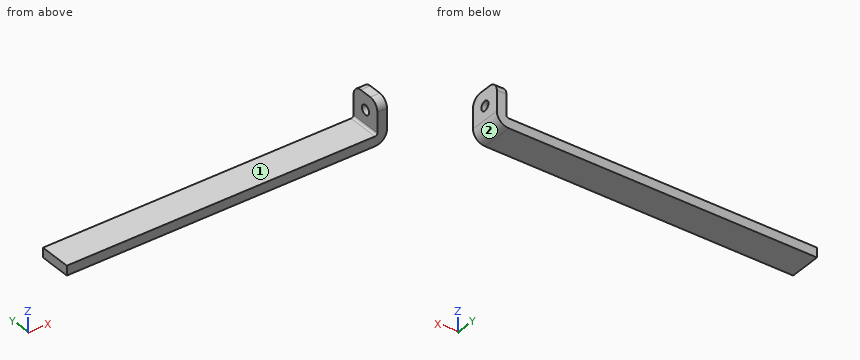
```python
from build123d import *

# Parameters (mm, degrees)
SKETCH_1_W                       = 100
SKETCH_1_H                       = 10
SM_BASE_FLANGE_1_DEPTH           = 3
SM_EDGE_FLANGE_1_STRIP_W         = 13.4732
SM_EDGE_FLANGE_1_STRIP_H         = 3
SM_EDGE_FLANGE_1_STRIP_CUT_DEPTH = 10
SM_EDGE_FLANGE_1_DEPTH           = 10
SKETCH_9_R                       = 1.5
CUT_EXTRUDE_1_DEPTH              = 10
FILLET_1_R                       = 3


# Sheet-metal steps are written as plain solids
with BuildPart() as part:
    # Sketch 1 → 基体-法兰1 (new body)
    with BuildSketch(Plane.XY):
        Rectangle(SKETCH_1_W, SKETCH_1_H)
    extrude(amount=-SM_BASE_FLANGE_1_DEPTH)

    # 边线-法兰1 strip (across the edge) → 边线-法兰1 strip cut (cut)
    with BuildSketch(Plane(origin=(50, -5, 0), x_dir=(-1, 0, 0), z_dir=(0, 1, 0))):
        with Locations((-3, -1.5)):
            Rectangle(SM_EDGE_FLANGE_1_STRIP_W, SM_EDGE_FLANGE_1_STRIP_H)
    extrude(amount=SM_EDGE_FLANGE_1_STRIP_CUT_DEPTH, mode=Mode.SUBTRACT)

    # 边线-法兰1 section (across the edge) → 边线-法兰1 (add)
    with BuildSketch(Plane(origin=(50, -5, 0), x_dir=(-1, 0, 0), z_dir=(0, 1, 0))):
        with BuildLine():
            Line((0, 0.7366), (0, 10))
            Line((0, 10), (3, 10))
            Line((3, 10), (3, 0.7366))
            ThreePointArc((3, 0.7366), (3.215745145, 0.215745145), (3.7366, 0))
            Line((3.7366, 0), (3.7366, -3))
            ThreePointArc((3.7366, -3), (1.094424801, -1.905575199), (0, 0.7366))
        make_face()
    extrude(amount=SM_EDGE_FLANGE_1_DEPTH)

    # 草图9 → 切除-拉伸1 (cut)
    with BuildSketch(Plane(origin=(50, 0, 0), x_dir=(0, 0, -1), z_dir=(1, 0, 0))):
        with Locations((-5, 0)):
            Circle(SKETCH_9_R)
    extrude(amount=-CUT_EXTRUDE_1_DEPTH, mode=Mode.SUBTRACT)

    # 圆角1
    fillet_1_edges = [part.edges().sort_by_distance(p)[0] for p in [
        (48.5, -5, 10),
        (48.5, 5, 10),
    ]]
    fillet(fillet_1_edges, radius=FILLET_1_R)


solid = part.part
```
Geometry: final body of the model. Coordinates: model frame, mm. Face numbers are marked on the shaded views. Round coordinates to 2 decimals unless told otherwise and drop trailing zeros. Write each loop counter-clockwise with the first axis right and the second up, starting at its lowest first coordinate (ties: lowest second). Pieces come first, ordered by that corner, then holes. Notation, with made-up numbers: M 23,40.5 L 69,40.5 A23 ccw 69,59.5 Z; hole C 30,21.5 d10. An arc over 180 degrees is marked long. Answer in a Markdown table with one row per item. Add a question column.
(1) Cut plane C-C, the plane x = -16.5. Return the cut outline in (y, z), then the cut area to 3 significant figures.
(2) Cut plane D-D, the plane y = -3.75. Return the cut outline in (x, z).
(3) Ray query, L1, parallel to Y at x = 48.45, z = 5; L2, parallel to X at y = -0.25, z = 7; L3, parallel to Z at x = 30, y = 4.25. Return the intervals inside material, ascending.
(4) Cut plane A-A, the plane z = 5. Return the cut outline in (x, y), then the cut area to 3 significant figures.
(5) Draft query along Z for the marked faces 1 and 2. Return one class per face: pulls with the +Z half, pulls with the -Z half, needs draft (parallel to the pull), parting line crosses it, or undercut.
(6) Contact query for flat-ended pins moving along their axis: pin 1 (2 mm diameter, centred on y = 0, z = 2, fed in from -X); pin 2 (6 mm diameter, centred on x = 9.5, y = 0.5, fed in from +Z); pin 3 (2 mm diameter, centred on x = -8.5, z = 2.5, fed in from +Y). Output: stop coordinate, or through.
(7) Cut plane B-B, the plane y = 0. Return the cut outline in (x, z).
Established:
| question | item | result |
|---|---|---|
| 1 | outline | M -5,-3 L 5,-3 L 5,0 L -5,0 Z |
| 1 | area | 30.0 mm² |
| 2 | outline | M -50,-3 L 46.26,-3 A3.74 ccw 50,0.74 L 50,9.44 L 47,9.44 L 47,0.74 A0.74 cw 46.26,0 L -50,0 Z |
| 3 | L1 | -5 to -1.5, 1.5 to 5 |
| 3 | L2 | 47 to 50 |
| 3 | L3 | -3 to 0 |
| 4 | outline | M 47,-5 L 50,-5 L 50,-1.5 L 47,-1.5 Z; M 47,1.5 L 50,1.5 L 50,5 L 47,5 Z |
| 4 | area | 21.0 mm² |
| 5 | face 1 | pulls with the +Z half |
| 5 | face 2 | pulls with the -Z half |
| 6 | pin 1 | x = 47 |
| 6 | pin 2 | z = 0 |
| 6 | pin 3 | through |
| 7 | outline | M -50,-3 L 46.26,-3 A3.74 ccw 50,0.74 L 50,3.5 L 47,3.5 L 47,0.74 A0.74 cw 46.26,0 L -50,0 Z; M 47,6.5 L 50,6.5 L 50,10 L 47,10 Z |
